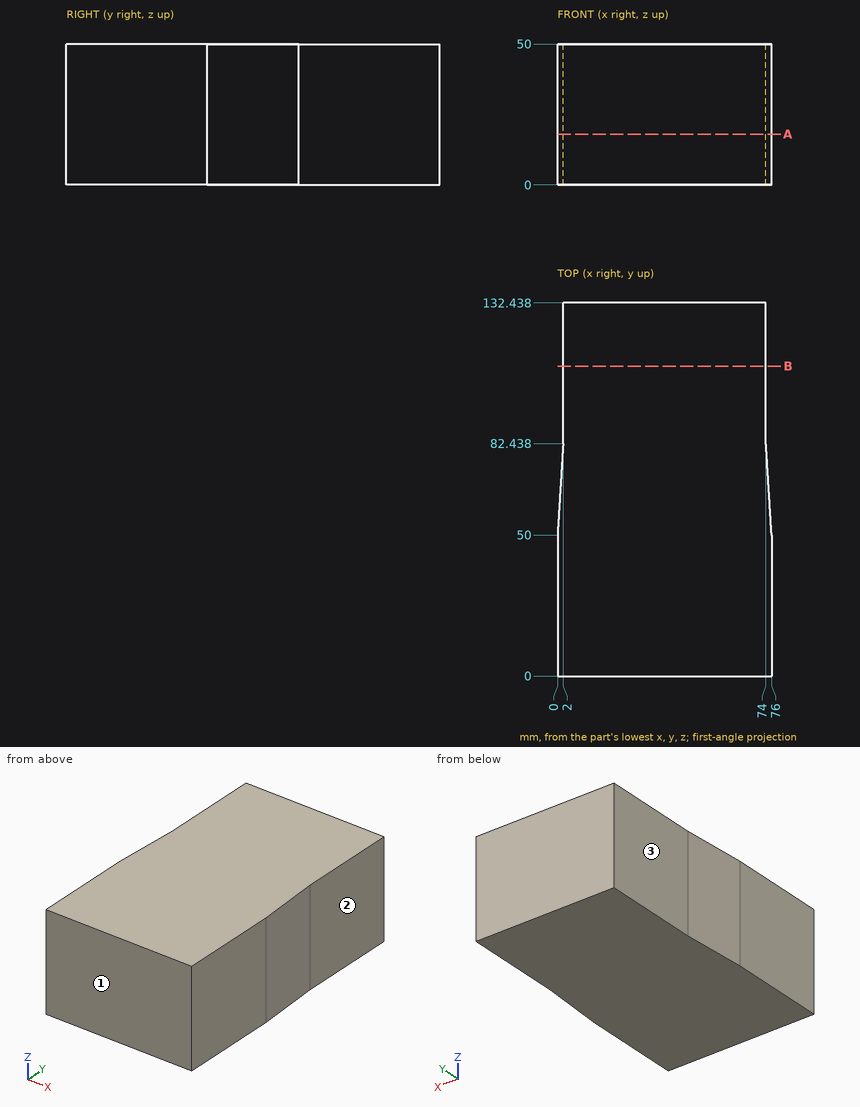
Here's the drawing with two shaded views (mm, measured from the low corner). I have some questions. A direction names the side the tool comes from. Coordinates: 2 decimals unless noted, no trailing zeros. Write each loop counter-clockwise with the first axis right and the second up, starting at its lowest first coordinate (ties: lowest second). Pieces come first, ordered by that corner, then holes. Notation, with made-up numbers: (64.25, 84) -> (123.25, 84) arc R21 ccw to (123.25, 108) -> close; hole circle Ø10 at (-4.75, -39). An arc over 180 degrees is marked (long way). Use a Markdown table: item, result. Add a question column.
(1) For the marked faces 1, 2 and 3, which set-ups out of +Z, -Z, +X, -X, +Y, -Y let a thin tool reach every point of the face, with its end or its side?
(2) If we section it at B-B, the plane y = 110: Write out the boundary of the cut face in (x, z), and give its area (3 significant figures).
(3) If we section it at A-A, the plane z = 18: Write out the boundary of the cut face in (x, y), and give its area (3 significant figures).
(4) I'm going to push flat-ended pins straight in: P1, Ø5, axis at x = 26, z = 29.5, coming from the -Y side; P2, Ø15, axis at y = 118, z = 19, coming from the -X side; P3, Ø25, axis at y = 104.5, z = 15.5, coming from the +X side; P4, Ø5, axis at y = 62, z = 25, coming from the -X side. Where does each tip first touch, or does it pass through?
(5) Please list where these lines run through material, in increasing order: line 1 (X direction, y = 100.5, z = 5); line 2 (X direction, y = 70.5, z = 15.5).
Outcome:
| question | item | result |
|---|---|---|
| 1 | face 1 | +Z, -Z, +X, -X, -Y |
| 1 | face 2 | +Z, -Z, +X, +Y |
| 1 | face 3 | +Z, -Z, -X, +Y |
| 2 | outline | (2, 0) -> (74, 0) -> (74, 50) -> (2, 50) -> close |
| 2 | area | 3,600 mm^2 |
| 3 | outline | (0, 0) -> (76, 0) -> (76, 50) -> (74, 82.44) -> (74, 132.44) -> (2, 132.44) -> (2, 82.44) -> (0, 50) -> close |
| 3 | area | 9,800 mm^2 |
| 4 | P1 | stops at y = 0 |
| 4 | P2 | stops at x = 2 |
| 4 | P3 | stops at x = 74 |
| 4 | P4 | stops at x = 0.59 |
| 5 | line 1 | x = 2 to 74 |
| 5 | line 2 | x = 1.26 to 74.74 |
